Answer from the drawing. Dimensions are ordinates in mm from the lowest x, y and z of the part. Round coordinates to 2 decimals unless told otherwise and drop trailing zeros. Loops run counter-clockwise (first coordinate to the right, second up) from the corner with the lowest first, then second, coordinate; pieces in that order, holes last. Notation, with made-up numbers: (54, 3.5) - (72, 3.5) arc R13 cw to (72, 13.5) - close; hole circle Ø1 at (-22, 5). An arc over 180 degrees is marked (long way). Answer as CSV lines item,"result". Start each with the question number.
Q1. Section A-A on y = 6 is taken. Write down the section's boundary in (x, z) (3 decimals).
Q2. Section B-B on z = 0.65 is taken. Write down the section's boundary in (x, y) (3 decimals).
Q3. Each of these flat-tipped pins is pushed along its axis until it touches: pin 1 Ø2 at (x, y) = (4.475, 6) entering from -Z; pin 2 Ø1.5 at (x, y) = (25, 10) entering from -Z. Where does it stop, or does it pass through?
Q4. Straight lines are drawn through the part: L1, parallel to X at y = 4.5, z = 0.6; L2, parallel to Y at x = 4, z = 0.65; L3, parallel to X at y = 7.25, z = 0.75. For each, find the intervals that lie inside material, in ascending order. Write a range as [from, to].
Q5. Section C-C on x = 24.5 is taken. Write down the section's boundary in (y, z), then the cut area to 3 significant figures.
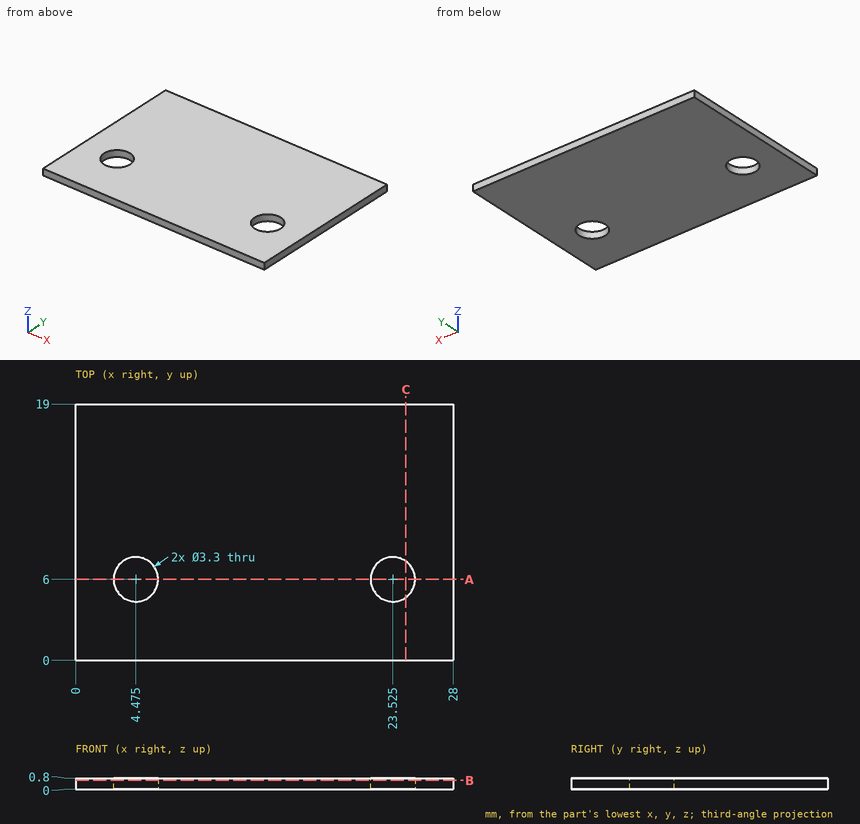
Findings:
1,outline,"(0, 0) - (2.825, 0) - (2.825, 0.8) - (0, 0.8) - close; (6.125, 0) - (21.875, 0) - (21.875, 0.8) - (6.125, 0.8) - close; (25.175, 0) - (28, 0) - (28, 0.8) - (25.175, 0.8) - close"
2,outline,"(0, 0) - (28, 0) - (28, 19) - (0, 19) - close; hole circle Ø3.3 at (4.475, 6); hole circle Ø3.3 at (23.525, 6)"
3,pin 1,"passes through"
3,pin 2,"stops at z = 0"
4,L1,"x = [0, 3.79], [5.16, 22.84], [24.21, 28]"
4,L2,"y = [0, 4.42], [7.58, 19]"
4,L3,"x = [0, 3.4], [5.55, 22.45], [24.6, 28]"
5,outline,"(0, 0) - (4.67, 0) - (4.67, 0.8) - (0, 0.8) - close; (7.33, 0) - (19, 0) - (19, 0.8) - (7.33, 0.8) - close"
5,area,"13.1 mm^2"
